The model under review builds one solid part; all positions refer to its coordinate system, in mm. Coordinates: 2 decimals unless noted, no trailing zeros. Order: outer loops, then holes, each group sorted by start corner. A loop starts at its lowest first (then second) coordinate and runs counter-clockwise, first axis right, second up. Notation, with made-up numbers: (-23, 81) -> (-7, 81) arc R26 ccw to (-7, 98) -> close; hole circle Ø10 at (69, 14.5). An arc over 180 degrees is marked (long way). Use one line per item in the form item = value.
Autodesk Inventor part; units mm, degrees
ref_plane "YZ Plane" through (0, 0, 0) normal (1, 0, 0) x (0, 1, 0)
ref_plane "XZ Plane" through (0, 0, 0) normal (0, 1, 0) x (-1, 0, 0)
ref_plane "XY Plane" through (0, 0, 0) normal (0, 0, 1) x (1, 0, 0)
sketch "スケッチ1" plane through (0, 0, 0) normal (0, 1, 0) x (-1, 0, 0)
  line L0 (0, 99) -> (30, 99)
  line L1 (30, 99) -> (30, -99)
  line L2 (30, -99) -> (0, -99)
  line L3 (0, -99) -> (0, 99)
  point P0 (0, 0)
  point P1 (0, 0)
  dimension "d0" = 198
  dimension "d1" = 30
extrude "押し出し1" add sketch "スケッチ1" along normal blind 2.5
sketch "スケッチ2" plane through (0, 2.5, 0) normal (0, 1, 0) x (1, 0, 0)
  line L0 (-30, 99) -> (-30, -99)
  line L1 (-30, -99) -> (-9, -99)
  line L2 (-9, -99) -> (-9, -59)
  line L3 (-9, -59) -> (-30, -59)
  line L4 (-30, -59) -> (-30, -99)
  point P0 (0, 0)
  dimension "d4" = 40
  dimension "d7" = 21
extrude "押し出し2" cut sketch "スケッチ2" against normal through all
mirror "ミラー1" about plane through (0, 0, 0) normal (0, 0, 1) of "押し出し2"
properties part number "front_upper" material "木材 (カエデ材)"
Item 1: We need section A-A (y = 1.95). Write out the cut boundary in (x, z), plus the area to 3 significant figures.
Results found:
outline = (-30, -59) -> (-9, -59) -> (-9, -99) -> (0, -99) -> (0, 99) -> (-9, 99) -> (-9, 59) -> (-30, 59) -> close
area = 4,260 mm²
Item 2: Clearance check with flat-ended pins moving along their axes: pin 1 (10 mm diameter, centred on x = -11.5, z = -34, fed in from -Y); pin 2 (0.8 mm diameter, centred on x = -24.5, y = 1.5, fed in from +Z); pin 3 (1.2 mm diameter, centred on x = -18.5, y = 1.5, fed in from -Z). State where each tip first meets the part, or that it passes through.
Results found:
pin_1 = 0
pin_2 = 59
pin_3 = -59
Item 3: To check wall thickness, follow L1, parallel to Z at x = -16.5, y = 0.1; L2, parallel to X at y = 1.8, z = -77. State the ranges of each line that lie inside material, in increasing order. Write a range as from..to.
Results found:
L1 = -59..59
L2 = -9..0
Item 4: We need section B-B (x = -16.75). Write out the cut boundary in (y, z), plus the area to 3 significant figures.
Results found:
outline = (0, -59) -> (2.5, -59) -> (2.5, 59) -> (0, 59) -> close
area = 295 mm²
Item 5: We need section C-C (z = -78). Write out the cut boundary in (x, y), plus the area to 3 significant figures.
Results found:
outline = (-9, 0) -> (0, 0) -> (0, 2.5) -> (-9, 2.5) -> close
area = 22.5 mm²
